Could you check a few things on this model? Use its own coordinates, in mm. A direction names the side the tool comes from. Coordinates: 2 decimals unless noted, no trailing zeros. Write each loop counter-clockwise with the first axis right and the second up, starting at its lowest first coordinate (ties: lowest second). Pieces come first, ordered by that corner, then holes.
Item 1: I want a section at B-B on z = 2.54. State how many separate pieces and enclosed holes the cut face has, then the cut area to 3 significant figures.
Item 2: Which directions (+Z, -Z, +X, -X, +Y, -Y) give clear straight access to the entire face, cutting with the end or side of a thin tool? Please do faces 1 (the cylindrical face through (12.71, -7.561, 3.554)), 2 (the flat face through (1, 2.632, 3)), 3 (the cylindrical face through (-7.063, 14.729, 3.346)).
Item 3: If I drill on probe 1 along Y at (x, z) = (18, 2.05); probe 2 along Z at (x, y) = (-18, 14.5); probe 3 along Y at (x, z) = (18.5, 1.6), over which ranges is the centre line in solid material (lowest first)?
Item 4: I want a section at A-A on y = 1. Please give me the cut outline in (x, z).
Item 5: For P1, Ø3, axis at x = 0, z = 3, coming from the +Y side; P2, Ø2.5, axis at x = 23.98, z = 2.54, coming from the +Y side; P3, Ø1, axis at x = 4, z = 3, coming from the -Y side; P4, Ø1, axis at x = 14.5, z = 3.5, coming from the +Y side, each with a flat end and sliding along its axis, tell me the tip position at first contact or that it passes through.
Item 6: Thinking about a two-plate mould opening in Z: for faces 4 (the flat face through (14.61, -0.487, 2.504)), 5 (the flat face through (3, 3, 0)), 6 (the cylindrical face through (-17, 14.75, 2.34)), which applies, +Z half, -Z half, draft (parallel to the pull), parting line (faces both ways), or undercut?
Item 7: I want a section at C-C on x = 0.5. Please give me the cut outline in (y, z).
Item 8: I want a section at D-D on y = 14. Please give me the cut outline in (x, z), then the cut area to 3 significant figures.
from build123d import *

# Parameters (mm, degrees)
BOSS_EXTRUDE1_DEPTH = 5.08
SKETCH2_R           = 1.5
CUT_EXTRUDE1_DEPTH  = 5.08
SKETCH3_R           = 1.5
CUT_EXTRUDE2_DEPTH  = 6.604


with BuildPart() as part:
    # Sketch1 → Boss-Extrude1 (new body)
    with BuildSketch(Plane.XY):
        Polygon((-22.656445993, 16.461324042), (-4.159581882, 16.461324042), (28.143554007, -8.938675958), (9.646689895, -8.938675958), align=None)
        Polygon((-13.356685139, 12.508658791), (-0.553226603, 2.631705063), (2.007465105, 2.631705063), (5.201047175, 6.771533672), (-2.806028737, 12.948420804), (-14.161473962, 12.948420804), align=None, mode=Mode.SUBTRACT)
        Polygon((2.017499691, -1.213937924), (8.409364086, -6.144804743), (21.944448825, -6.144804743), (7.067180743, 5.33194492), align=None, mode=Mode.SUBTRACT)
    extrude(amount=BOSS_EXTRUDE1_DEPTH)

    # Sketch2 → Cut-Extrude1 (cut)
    with BuildSketch(Plane(origin=(0, 16.461324042, 0), x_dir=(1, 0, 0), z_dir=(0, 1, 0))):
        with Locations(Location((-18.488013937, -2.54, 0), (0, 0, 270))):
            Circle(SKETCH2_R)
        with Locations(Location((-8.328013937, -2.54, 0), (0, 0, 270))):
            Circle(SKETCH2_R)
    extrude(amount=-CUT_EXTRUDE1_DEPTH, mode=Mode.SUBTRACT)

    # Sketch3 → Cut-Extrude2 (cut)
    with BuildSketch(Plane(origin=(0, -8.938675958, 0), x_dir=(-1, 0, 0), z_dir=(0, -1, 0))):
        with Locations(Location((-23.975121951, -2.54, 0), (0, 0, 180))):
            Circle(SKETCH3_R)
        with Locations(Location((-13.815121951, -2.54, 0), (0, 0, 180))):
            Circle(SKETCH3_R)
    extrude(amount=-CUT_EXTRUDE2_DEPTH, mode=Mode.SUBTRACT)


solid = part.part
Response values:
1. separate pieces: 3
1. enclosed holes: 0
1. area: 223 mm2
2. face 1: -Y
2. face 2: +Z, -Z
2. face 3: +Y
3. probe 1: y = -8.94 to -6.14, -3.1 to -0.96
3. probe 2: z = 0 to 1.12, 3.96 to 5.08
3. probe 3: y = -8.94 to -6.14, -3.49 to -1.36
4. outline: (-2.99, 0) - (3.73, 0) - (3.73, 5.08) - (-2.99, 5.08) - close; (12.68, 0) - (15.5, 0) - (15.5, 5.08) - (12.68, 5.08) - close
5. P1: stops at y = 14.37
5. P2: passes through
5. P3: stops at y = -4.89
5. P4: stops at y = 2.18
6. face 4: draft
6. face 5: -Z half
6. face 6: undercut
7. outline: (-1.75, 0) - (2.63, 0) - (2.63, 5.08) - (-1.75, 5.08) - close; (10.4, 0) - (12.8, 0) - (12.8, 5.08) - (10.4, 5.08) - close
8. outline: (-19.53, 0) - (-1.03, 0) - (-1.03, 5.08) - (-19.53, 5.08) - (-19.53, 3.62) arc R1.5 cw (long way) to (-19.53, 1.46) - close; hole circle Ø3 at (-8.33, 2.54)
8. area: 80.5 mm2
